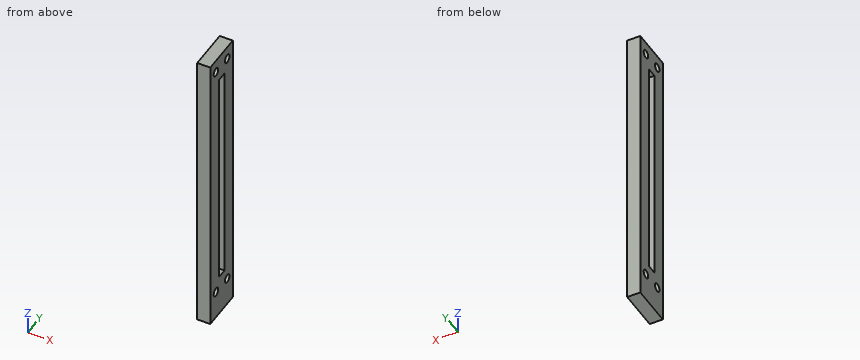
```python
from build123d import *

# Parameters (mm, degrees)
CYLINDER075_R           = 1.6
CYLINDER075_DEPTH       = 40
CYLINDER075_PITCH_ANGLE = 90
CYLINDER065_R           = 1.6
CYLINDER065_DEPTH       = 40
CYLINDER065_PITCH_ANGLE = 90
CYLINDER064_R           = 1.6
CYLINDER064_DEPTH       = 40
CYLINDER064_PITCH_ANGLE = 90
CYLINDER074_R           = 1.6
CYLINDER074_DEPTH       = 40
CYLINDER074_PITCH_ANGLE = 90
CYLINDER072_R           = 1.6
CYLINDER072_DEPTH       = 40
CYLINDER072_PITCH_ANGLE = 90
CYLINDER071_R           = 1.6
CYLINDER071_DEPTH       = 40
CYLINDER071_PITCH_ANGLE = 90
BOX021_W                = 10
BOX021_H                = 4
BOX021_DEPTH            = 86
BOX020_W                = 5
BOX020_H                = 16
BOX020_DEPTH            = 112


with BuildPart() as cylinder353:
    # Cylinder075 → Cylinder075 (new body)
    with BuildSketch(Plane.XY):
        Circle(CYLINDER075_R)
    extrude(amount=CYLINDER075_DEPTH)


with BuildPart() as cylinder353_1:
    # Cylinder075 pitch: moved
    add(cylinder353.part.rotate(Axis((0, 0, 0), (0, 1, 0)), CYLINDER075_PITCH_ANGLE))


with BuildPart() as cylinder353_2:
    # Cylinder075 placement: moved
    add(cylinder353_1.part.moved(Location((-67, 7, 126))))


with BuildPart() as cylinder343:
    # Cylinder065 → Cylinder065 (new body)
    with BuildSketch(Plane.XY):
        Circle(CYLINDER065_R)
    extrude(amount=CYLINDER065_DEPTH)


with BuildPart() as cylinder343_1:
    # Cylinder065 pitch: moved
    add(cylinder343.part.rotate(Axis((0, 0, 0), (0, 1, 0)), CYLINDER065_PITCH_ANGLE))


with BuildPart() as cylinder343_2:
    # Cylinder065 placement: moved
    add(cylinder343_1.part.moved(Location((-67, -15, 30))))


with BuildPart() as rocker_screw_holes_d:
    # Cylinder064 → Cylinder064 (new body)
    with BuildSketch(Plane.XY):
        Circle(CYLINDER064_R)
    extrude(amount=CYLINDER064_DEPTH)


with BuildPart() as rocker_screw_holes_d_1:
    # Cylinder064 pitch: moved
    add(rocker_screw_holes_d.part.rotate(Axis((0, 0, 0), (0, 1, 0)), CYLINDER064_PITCH_ANGLE))


with BuildPart() as rocker_screw_holes_d_2:
    # Cylinder064 placement: moved
    add(rocker_screw_holes_d_1.part.moved(Location((-87, -7, 30))))

    # Fusion042: union Cylinder343
    add(cylinder343_2.part)


with BuildPart() as rocker_screw_holes_d_3:
    # Fusion042 placement: moved
    add(rocker_screw_holes_d_2.part.moved(Location((0, 0, 96))))

    # Fusion050: union Cylinder353
    add(cylinder353_2.part)


with BuildPart() as cylinder352:
    # Cylinder074 → Cylinder074 (new body)
    with BuildSketch(Plane.XY):
        Circle(CYLINDER074_R)
    extrude(amount=CYLINDER074_DEPTH)


with BuildPart() as cylinder352_1:
    # Cylinder074 pitch: moved
    add(cylinder352.part.rotate(Axis((0, 0, 0), (0, 1, 0)), CYLINDER074_PITCH_ANGLE))


with BuildPart() as cylinder352_2:
    # Cylinder074 placement: moved
    add(cylinder352_1.part.moved(Location((-67, 7, 30))))


with BuildPart() as cylinder350:
    # Cylinder072 → Cylinder072 (new body)
    with BuildSketch(Plane.XY):
        Circle(CYLINDER072_R)
    extrude(amount=CYLINDER072_DEPTH)


with BuildPart() as cylinder350_1:
    # Cylinder072 pitch: moved
    add(cylinder350.part.rotate(Axis((0, 0, 0), (0, 1, 0)), CYLINDER072_PITCH_ANGLE))


with BuildPart() as cylinder350_2:
    # Cylinder072 placement: moved
    add(cylinder350_1.part.moved(Location((-67, -15, 30))))


with BuildPart() as rocker_screw_holes_c:
    # Cylinder071 → Cylinder071 (new body)
    with BuildSketch(Plane.XY):
        Circle(CYLINDER071_R)
    extrude(amount=CYLINDER071_DEPTH)


with BuildPart() as rocker_screw_holes_c_1:
    # Cylinder071 pitch: moved
    add(rocker_screw_holes_c.part.rotate(Axis((0, 0, 0), (0, 1, 0)), CYLINDER071_PITCH_ANGLE))


with BuildPart() as rocker_screw_holes_c_2:
    # Cylinder071 placement: moved
    add(rocker_screw_holes_c_1.part.moved(Location((-87, -7, 30))))

    # Fusion047: union Cylinder350
    add(cylinder350_2.part)

    # Fusion049: union Cylinder352
    add(cylinder352_2.part)


with BuildPart() as string_hole001:
    # Box021 → Box021 (new body)
    with BuildSketch(Plane(origin=(-46, -13, 35), x_dir=(1, 0, 0), z_dir=(0, 0, 1))):
        with Locations((5, 2)):
            Rectangle(BOX021_W, BOX021_H)
    extrude(amount=BOX021_DEPTH)


with BuildPart() as string_slot_c:
    # Box020 → Box020 (new body)
    with BuildSketch(Plane(origin=(-43, -19, 19), x_dir=(1, 0, 0), z_dir=(0, 0, 1))):
        with Locations((2.5, 8)):
            Rectangle(BOX020_W, BOX020_H)
    extrude(amount=BOX020_DEPTH)

    # Cut031: cut string-hole001
    add(string_hole001.part, mode=Mode.SUBTRACT)


with BuildPart() as string_slot_c_1:
    # Cut031 placement: moved
    add(string_slot_c.part.moved(Location((-11, 0, 0))))

    # Cut041: cut rocker-screw-holes-c
    add(rocker_screw_holes_c_2.part, mode=Mode.SUBTRACT)

    # Cut042: cut rocker-screw-holes-d
    add(rocker_screw_holes_d_3.part, mode=Mode.SUBTRACT)


solid = string_slot_c_1.part
```
Can you work these out from the model? Positions are in its coordinate system, mm. Coordinates: 2 decimals unless noted, no trailing zeros. Write each loop counter-clockwise with the first axis right and the second up, starting at its lowest first coordinate (ties: lowest second). Pieces come first, ordered by that corner, then holes. Notation, with made-up numbers: M 52.25,87 L 109.25,87 A28 cw 109.25,126 Z; hole C -30,-23 d8. An arc over 180 degrees is marked long. Answer as CSV lines item,"result".
Item 1: Imagine slicing it at A-A on z = 109. List the corners of the cut face in (x, y) for me.
Geometry results:
outline,"M -54,-19 L -49,-19 L -49,-13 L -54,-13 Z; M -54,-9 L -49,-9 L -49,-3 L -54,-3 Z"
Item 2: Imagine slicing it at B-B on y = -7. List the corners of the cut face in (x, z) for me, plus the area to 3 significant figures.
Geometry results:
outline,"M -54,19 L -49,19 L -49,28.4 L -54,28.4 Z; M -54,31.6 L -49,31.6 L -49,124.4 L -54,124.4 Z; M -54,127.6 L -49,127.6 L -49,131 L -54,131 Z"
area,"528 mm2"
Item 3: Imagine slicing it at C-C on x = -52.2. List the corners of the cut face in (y, z) for me, plus the area to 3 significant figures.
Geometry results:
outline,"M -19,19 L -3,19 L -3,131 L -19,131 Z; hole C -15,30 d3.2; hole C -15,126 d3.2; hole M -13,35 L -9,35 L -9,121 L -13,121 Z; hole C -7,30 d3.2; hole C -7,126 d3.2"
area,"1,420 mm2"
Item 4: Please list where these lines run through material, in increasing order: line 1 along Y through (x, z) = (-52.9, 126); line 2 along Z through (x, y) = (-50, -7); line 3 along Y through (x, z) = (-52.1, 76.5).
Geometry results:
line 1,"y = -19 to -16.6, -13.4 to -8.6, -5.4 to -3"
line 2,"z = 19 to 28.4, 31.6 to 124.4, 127.6 to 131"
line 3,"y = -19 to -13, -9 to -3"
Item 5: Imagine slicing it at D-D on z = 30. List the corners of the cut face in (x, y) for me, plus the area to 3 significant figures.
Geometry results:
outline,"M -54,-19 L -49,-19 L -49,-16.6 L -54,-16.6 Z; M -54,-13.4 L -49,-13.4 L -49,-8.6 L -54,-8.6 Z; M -54,-5.4 L -49,-5.4 L -49,-3 L -54,-3 Z"
area,"48.0 mm2"
